CAD build for the part. Positions are in the model's coordinates, mm. A direction names the side the tool comes from. Give positions to 0.01 mm unless a question says otherwise; leave off trailing zeros. Write each loop counter-clockwise with the first axis right and the second up, starting at its lowest first coordinate (ties: lowest second). Pieces come first, ordered by that corner, then holes. Notation, with made-up numbers: (-29, 52) - (-18, 52) arc R24 cw to (-18, 70) - close; hole circle Ø10 at (23, 79.25). An arc over 180 degrees is marked (long way). Put each result on its own line as item: value. Start each with the question number.
1. Cut at B-B on x = 29.5. List the corners of the cut face in (y, z), and give its area (3 significant figures).
2. Drop flat-ended pins along their axis: pin 1 (8 mm diameter, centred on x = 6.5, y = 12, fed in from +Z); pin 2 (8 mm diameter, centred on y = 45.5, z = 13, fed in from -X); pin 3 (4 mm diameter, centred on x = 39, z = 10, fed in from +Y); pin 4 (7 mm diameter, centred on y = 28.5, z = 8, fed in from +X). Give the stop position or say it passes through.
3. Cut at D-D on x = 35.5. List the corners of the cut face in (y, z).
4. Tool access for faces 4 (the flat face through (2, 26.22, 17)), 5 (the flat face through (2, 21.22, 17)), 6 (the flat face through (4, 31, 6)), 7 (the flat face through (24, 2, 2.284)): list every direction of +Z, -Z, +X, -X, +Y, -Y with a clear straight run to the whole face (end or side of a thin tool).
5. Cut at A-A on z = 16.25. List the corners of the cut face in (x, y), and give its area (3 significant figures).
6. Wall check: line 1 (Y direction, x = 1.1, z = 16.25); line 2 (X direction, y = 33, z = 9). Give the ranges that are in metal, low to high.
7. Cut at C-C on y = 23.72. List the corners of the cut face in (x, z).
8. Mould opens along Z. For faces 1 (the cylindrical face through (25.52, 2.03, 6.92)), 2 (the flat face through (2, 49, 17)), 3 (the flat face through (2, 15, 0)) say: +Z half, -Z half, draft (parallel to the pull), parting line (faces both ways), or undercut.
from build123d import *

# Parameters (mm, degrees)
SKETCH_1_W          = 4
SKETCH_1_H          = 50
SKETCH_1_W_2        = 45
SKETCH_1_H_2        = 4
EXTRUDE_1_DEPTH     = 10
SKETCH_2_W          = 4
SKETCH_2_H          = 5
EXTRUDE_2_DEPTH     = 12.5
SKETCH_3_R          = 1
CUT_EXTRUDE_1_DEPTH = 4
FILLET_1_DEPTH      = 10
FILLET_2_SIZE       = 4
FILLET_3_SIZE       = 2
FILLET_4_SIZE       = 2
SKETCH_27_R         = 1.552273675
CUT_EXTRUDE_2_DEPTH = 4
CUT_EXTRUDE_2_DRAFT = -7.86
FILLET_5_R          = 2
FILLET_6_R          = 2
FILLET_7_R          = 2
SKETCH_32_W         = 17.415964898
SKETCH_32_H         = 1.123035165
CUT_EXTRUDE_3_DEPTH = 4
SKETCH_26_R         = 2.45
CUT_EXTRUDE3_DEPTH  = 10
FILLET1_R           = 0.5
FILLET2_R           = 0.5
FILLET3_R           = 0.5
FILLET4_R           = 0.5


with BuildPart() as part:
    # Эскиз1 → Бобышка-Вытянуть1 (new body)
    with BuildSketch(Plane.XY):
        with Locations((2, 29)):
            Rectangle(SKETCH_1_W, SKETCH_1_H)
        with Locations((22.5, 2)):
            Rectangle(SKETCH_1_W_2, SKETCH_1_H_2)
    extrude(amount=EXTRUDE_1_DEPTH)

    # Эскиз2 → Бобышка-Вытянуть2 (add)
    with BuildSketch(Plane.XY.offset(10)):
        with Locations((2, 51.5)):
            Rectangle(SKETCH_2_W, SKETCH_2_H)
        with Locations((2, 23.72)):
            Rectangle(SKETCH_2_W, SKETCH_2_H)
    extrude(amount=EXTRUDE_2_DEPTH)

    # Эскиз3 → Вырез-Вытянуть1 (cut)
    with BuildSketch(Plane(origin=(4, 0, 0), x_dir=(0, 0, -1), z_dir=(1, 0, 0))):
        with Locations((-16.25, 51.5)):
            Circle(SKETCH_3_R)
        with Locations((-16.25, 23.72)):
            Circle(SKETCH_3_R)
    extrude(amount=-CUT_EXTRUDE_1_DEPTH, mode=Mode.SUBTRACT)

    # Скругление1: read off the stored shape, not the designer's step
    # Скругление1 outline → Скругление1 (add)
    with BuildSketch(Plane.XY):
        with BuildLine():
            Line((4, 4), (8, 4))
            add(Edge.make_bspline(
                [(8, 4), (4, 4), (4, 8)],
                knots=[0, 0, 0, 1, 1, 1], degree=2))
            Line((4, 8), (4, 4))
        make_face()
    extrude(amount=FILLET_1_DEPTH)

    # Скругление2
    # a fillet whose section is not a circle: 4 mm, written as the material it takes off along each edge
    with BuildSketch(Plane(origin=(0, 0, -10), x_dir=(0, 1, 0), z_dir=(0, 0, 1))) as fillet_2_piece_1:
        with BuildLine():
            Bezier((FILLET_2_SIZE, 0), (0, 0), (0, -FILLET_2_SIZE), weights=[1, 1, 1])
            Line((0, -FILLET_2_SIZE), (0, 0))
            Line((0, 0), (FILLET_2_SIZE, 0))
        make_face()
    extrude(amount=30, mode=Mode.SUBTRACT)

    # Скругление3
    # a fillet whose section is not a circle: 2 mm, written as the material it takes off along each edge
    with BuildSketch(Plane(origin=(45, 4, -5), x_dir=(-1, 0, 0), z_dir=(0, 0, 1))) as fillet_3_piece_1:
        with BuildLine():
            Bezier((FILLET_3_SIZE, 0), (0, 0), (0, FILLET_3_SIZE), weights=[1, 1, 1])
            Line((0, FILLET_3_SIZE), (0, 0))
            Line((0, 0), (FILLET_3_SIZE, 0))
        make_face()
    extrude(amount=20, mode=Mode.SUBTRACT)

    # Скругление4
    # a fillet whose section is not a circle: 2 mm, written as the material it takes off along each edge
    with BuildSketch(Plane(origin=(45, 0, -5), x_dir=(0, 1, 0), z_dir=(0, 0, 1))) as fillet_4_piece_1:
        with BuildLine():
            Bezier((FILLET_4_SIZE, 0), (0, 0), (0, FILLET_4_SIZE), weights=[1, 1, 1])
            Line((0, FILLET_4_SIZE), (0, 0))
            Line((0, 0), (FILLET_4_SIZE, 0))
        make_face()
    extrude(amount=20, mode=Mode.SUBTRACT)


with BuildPart() as cut_extrude_2_tool:
    # Эскиз27 → Вырез-Вытянуть2 (with draft: the straight prism first)
    with BuildSketch(Plane(origin=(0, 4, 0), x_dir=(1, 0, 0), z_dir=(0, 1, 0))):
        with Locations((23.455175104, -5.602717063)):
            Circle(SKETCH_27_R)
    extrude(amount=-CUT_EXTRUDE_2_DEPTH)
    # Вырез-Вытянуть2: the draft: its side faces are tilted about the plane it starts from
    cut_extrude_2_sides = [cut_extrude_2_tool.faces().sort_by_distance(p)[0] for p in [
        (21.902901429, 2, 5.602717063),
    ]]
    draft(cut_extrude_2_sides, Plane(origin=(0, 4, 0), x_dir=(1, 0, 0), z_dir=(0, 1, 0)), CUT_EXTRUDE_2_DRAFT)


with BuildPart() as part_1:
    add(part.part)

    # Вырез-Вытянуть2: cut by cut_extrude_2_tool
    add(cut_extrude_2_tool.part, mode=Mode.SUBTRACT)

    # Скругление5
    fillet_5_edges = [part_1.edges().sort_by_distance(p)[0] for p in [
        (2, 49, 10),
    ]]
    fillet(fillet_5_edges, radius=FILLET_5_R)

    # Скругление6
    fillet_6_edges = [part_1.edges().sort_by_distance(p)[0] for p in [
        (2, 21.22, 10),
    ]]
    fillet(fillet_6_edges, radius=FILLET_6_R)

    # Скругление7
    fillet_7_edges = [part_1.edges().sort_by_distance(p)[0] for p in [
        (2, 26.22, 10),
    ]]
    fillet(fillet_7_edges, radius=FILLET_7_R)

    # Эскиз32 → Вырез-Вытянуть3 (cut)
    with BuildSketch(Plane(origin=(0, 4, 0), x_dir=(1, 0, 0), z_dir=(0, 1, 0))):
        with Locations((23.917887929, -1.722044793)):
            Rectangle(SKETCH_32_W, SKETCH_32_H)
    extrude(amount=-CUT_EXTRUDE_3_DEPTH, mode=Mode.SUBTRACT)

    # Эскиз26 → Cut-Extrude3 (cut)
    with BuildSketch(Plane(origin=(0, 4, 0), x_dir=(1, 0, 0), z_dir=(0, 1, 0))):
        with Locations(Location((23.455175104, -5.602717063, 0), (0, 0, 270))):
            Circle(SKETCH_26_R)
    extrude(amount=-CUT_EXTRUDE3_DEPTH, mode=Mode.SUBTRACT)

    # Fillet1
    fillet1_edges = [part_1.edges().sort_by_distance(p)[0] for p in [
        (32.625870378, 2, 1.16052721),
    ]]
    fillet(fillet1_edges, radius=FILLET1_R)

    # Fillet2
    fillet2_edges = [part_1.edges().sort_by_distance(p)[0] for p in [
        (32.625870378, 2, 2.283562375),
    ]]
    fillet(fillet2_edges, radius=FILLET2_R)

    # Fillet3
    fillet3_edges = [part_1.edges().sort_by_distance(p)[0] for p in [
        (15.20990548, 2, 1.16052721),
    ]]
    fillet(fillet3_edges, radius=FILLET3_R)

    # Fillet4
    fillet4_edges = [part_1.edges().sort_by_distance(p)[0] for p in [
        (15.20990548, 2, 2.283562375),
    ]]
    fillet(fillet4_edges, radius=FILLET4_R)


solid = part_1.part
Report:
1. outline: (0, 0) - (4, 0) - (4, 1.16) - (0, 1.16) - close; (0, 2.28) - (4, 2.28) - (4, 10) - (0, 10) - close
1. area: 35.5 mm²
2. pin 1: stops at z = 10
2. pin 2: stops at x = 0
2. pin 3: stops at y = 4
2. pin 4: stops at x = 4
3. outline: (0, 0) - (4, 0) - (4, 10) - (0, 10) - close
4. face 4: +Z, +X, -X
4. face 5: +Z, +X, -X, -Y
4. face 6: +Z, -Z, +X, +Y
4. face 7: +Y, -Y
5. outline: (0, 21.22) - (4, 21.22) - (4, 22.72) - (0, 22.72) - close; (0, 24.72) - (4, 24.72) - (4, 26.22) - (0, 26.22) - close; (0, 49) - (4, 49) - (4, 50.5) - (0, 50.5) - close; (0, 52.5) - (4, 52.5) - (4, 54) - (0, 54) - close
5. area: 24.0 mm²
6. line 1: y = 21.22 to 22.72, 24.72 to 26.22, 49 to 50.5, 52.5 to 54
6. line 2: x = 0 to 4
7. outline: (0, 0) - (4, 0) - (4, 15.25) - (0, 15.25) - close; (0, 17.25) - (4, 17.25) - (4, 22.5) - (0, 22.5) - close
8. face 1: undercut
8. face 2: draft
8. face 3: -Z half
